from build123d import *

# Parameters (mm, degrees)
CROQUIS1_W              = 102
CROQUIS1_H              = 50
SALIENTE_EXTRUIR1_DEPTH = 40
CORTAR_EXTRUIR1_DEPTH   = 38
CROQUIS4_R              = 2
CORTAR_EXTRUIR2_DEPTH   = 18
CORTAR_EXTRUIR3_DEPTH   = 38
CROQUIS7_W              = 6
CROQUIS7_H              = 3
CORTAR_EXTRUIR5_DEPTH   = 10
SALIENTE_EXTRUIR2_DEPTH = 5
CROQUIS9_W              = 6
CROQUIS9_H              = 1
SALIENTE_EXTRUIR3_DEPTH = 3
REDONDEO2_R             = 2
REDONDEO4_R             = 2
CROQUIS16_W             = 36.5
CROQUIS16_H             = 26.972151698
CORTAR_EXTRUIR13_DEPTH  = 5.5
CROQUIS17_W             = 40
CROQUIS17_H             = 30
CROQUIS17_W_2           = 36.5
CROQUIS17_H_2           = 26.972151698
SALIENTE_EXTRUIR7_DEPTH = 13.5
CROQUIS18_W             = 1.5
CROQUIS18_H             = 36.5
SALIENTE_EXTRUIR8_DEPTH = 27.5
CROQUIS19_R             = 11
CORTAR_EXTRUIR14_DEPTH  = 27.5
REDONDEO5_R             = 2


with BuildPart() as part:
    # Croquis1 → Saliente-Extruir1 (new body)
    with BuildSketch(Plane.XY):
        Rectangle(CROQUIS1_W, CROQUIS1_H)
    extrude(amount=SALIENTE_EXTRUIR1_DEPTH)

    # Croquis3 → Cortar-Extruir1 (cut)
    with BuildSketch(Plane.XY.offset(40)):
        with BuildLine():
            Line((51, 25), (41, 25))
            Line((41, 25), (41, 18))
            ThreePointArc((41, 18), (41.878679656, 15.878679656), (44, 15))
            Line((44, 15), (51, 15))
            Line((51, 15), (51, 25))
        make_face()
        with BuildLine():
            Line((41, -18), (41, -25))
            Line((41, -25), (51, -25))
            Line((51, -25), (51, -15))
            Line((51, -15), (44, -15))
            ThreePointArc((44, -15), (41.878679656, -15.878679656), (41, -18))
        make_face()
        with BuildLine():
            Line((-44, -15), (-51, -15))
            Line((-51, -15), (-51, -25))
            Line((-51, -25), (-41, -25))
            Line((-41, -25), (-41, -18))
            ThreePointArc((-41, -18), (-41.878679656, -15.878679656), (-44, -15))
        make_face()
        with BuildLine():
            Line((-51, 25), (-51, 15))
            Line((-51, 15), (-44, 15))
            ThreePointArc((-44, 15), (-41.878679656, 15.878679656), (-41, 18))
            Line((-41, 18), (-41, 25))
            Line((-41, 25), (-51, 25))
        make_face()
    extrude(amount=-CORTAR_EXTRUIR1_DEPTH, mode=Mode.SUBTRACT)

    # Croquis4 → Cortar-Extruir2 (cut)
    with BuildSketch(Plane.XY.offset(2)):
        with BuildLine():
            Line((-51, -25), (-48, -25))
            ThreePointArc((-48, -25), (-50.121320344, -24.121320344), (-51, -22))
            Line((-51, -22), (-51, -25))
        make_face()
        with Locations((-46, -20)):
            Circle(CROQUIS4_R)
        with BuildLine():
            Line((-51, 25), (-51, 22))
            ThreePointArc((-51, 22), (-50.121320344, 24.121320344), (-48, 25))
            Line((-48, 25), (-51, 25))
        make_face()
        with Locations((-46, 20)):
            Circle(CROQUIS4_R)
        with Locations((46, 20)):
            Circle(CROQUIS4_R)
        with BuildLine():
            ThreePointArc((48, 25), (50.121320344, 24.121320344), (51, 22))
            Line((51, 22), (51, 25))
            Line((51, 25), (48, 25))
        make_face()
        with Locations((46, -20)):
            Circle(CROQUIS4_R)
        with BuildLine():
            ThreePointArc((51, -22), (50.121320344, -24.121320344), (48, -25))
            Line((48, -25), (51, -25))
            Line((51, -25), (51, -22))
        make_face()
    extrude(amount=-CORTAR_EXTRUIR2_DEPTH, mode=Mode.SUBTRACT)

    # Croquis5 → Cortar-Extruir3 (cut)
    with BuildSketch(Plane(origin=(0, 0, 0), x_dir=(-1, 0, 0), z_dir=(0, 0, -1))):
        with BuildLine():
            Line((0, 23.5), (-39.490487895, 23.5))
            Line((-39.490487895, 23.5), (-39.490487895, 15.5))
            ThreePointArc((-39.490487895, 15.5), (-40.076274332, 14.085786438), (-41.490487895, 13.5))
            Line((-41.490487895, 13.5), (-49.525351845, 13.5))
            Line((-49.525351845, 13.5), (-49.525351845, -13.472151698))
            Line((-49.525351845, -13.472151698), (-41.490487895, -13.472151698))
            ThreePointArc((-41.490487895, -13.472151698), (-40.076274332, -14.057938136), (-39.490487895, -15.472151698))
            Line((-39.490487895, -15.472151698), (-39.490487895, -23.5))
            Line((-39.490487895, -23.5), (39.5, -23.5))
            Line((39.5, -23.5), (39.5, -15.472151698))
            ThreePointArc((39.5, -15.472151698), (40.085786438, -14.057938136), (41.5, -13.472151698))
            Line((41.5, -13.472151698), (49.474648155, -13.472151698))
            Line((49.474648155, -13.472151698), (49.474648155, 13.5))
            Line((49.474648155, 13.5), (41.5, 13.5))
            ThreePointArc((41.5, 13.5), (40.085786438, 14.085786438), (39.5, 15.5))
            Line((39.5, 15.5), (39.5, 23.5))
            Line((39.5, 23.5), (0, 23.5))
        make_face()
    extrude(amount=-CORTAR_EXTRUIR3_DEPTH, mode=Mode.SUBTRACT)

    # Croquis7 → Cortar-Extruir5 (cut)
    with BuildSketch(Plane(origin=(0, 25, 0), x_dir=(1, 0, 0), z_dir=(0, 1, 0))):
        with Locations((0, -1.5)):
            Rectangle(CROQUIS7_W, CROQUIS7_H)
    extrude(amount=-CORTAR_EXTRUIR5_DEPTH, mode=Mode.SUBTRACT)

    # Croquis8 → Saliente-Extruir2 (add)
    with BuildSketch(Plane(origin=(0, 25, 0), x_dir=(1, 0, 0), z_dir=(0, 1, 0))):
        Polygon((3, 0), (4, 0), (4, -4), (-4, -4), (-4, 0), (-3, 0), (-3, -3), (3, -3), align=None)
    extrude(amount=SALIENTE_EXTRUIR2_DEPTH)

    # Croquis9 → Saliente-Extruir3 (add)
    with BuildSketch(Plane(origin=(0, 0, 3), x_dir=(-1, 0, 0), z_dir=(0, 0, -1))):
        with Locations((0, 29.5)):
            Rectangle(CROQUIS9_W, CROQUIS9_H)
    extrude(amount=SALIENTE_EXTRUIR3_DEPTH)

    # Redondeo2
    redondeo2_edges = [part.edges().sort_by_distance(p)[0] for p in [
        (0, 23.5, 3),
    ]]
    fillet(redondeo2_edges, radius=REDONDEO2_R)

    # Redondeo4
    redondeo4_edges = [part.edges().sort_by_distance(p)[0] for p in [
        (-4, 25, 2),
        (0, 25, 4),
        (4, 25, 2),
    ]]
    fillet(redondeo4_edges, radius=REDONDEO4_R)

    # Croquis16 → Cortar-Extruir13 (cut)
    with BuildSketch(Plane(origin=(-49.474648155, 0, 0), x_dir=(0, 0, -1), z_dir=(1, 0, 0))):
        with Locations((-19.75, 0.013924151)):
            Rectangle(CROQUIS16_W, CROQUIS16_H)
    extrude(amount=-CORTAR_EXTRUIR13_DEPTH, mode=Mode.SUBTRACT)

    # Croquis17 → Saliente-Extruir7 (add)
    with BuildSketch(Plane.ZY.offset(51)):
        with Locations((20, 0)):
            Rectangle(CROQUIS17_W, CROQUIS17_H)
        with Locations((19.75, 0.013924151)):
            Rectangle(CROQUIS17_W_2, CROQUIS17_H_2, mode=Mode.SUBTRACT)
    extrude(amount=SALIENTE_EXTRUIR7_DEPTH)

    # Croquis18 → Saliente-Extruir8 (add)
    with BuildSketch(Plane.XZ.offset(-13.5)):
        with Locations((-63.75, 19.75)):
            Rectangle(CROQUIS18_W, CROQUIS18_H)
    extrude(amount=SALIENTE_EXTRUIR8_DEPTH)

    # Croquis19 → Cortar-Extruir14 (cut)
    with BuildSketch(Plane.ZY.offset(64.5)):
        with Locations((20, 0)):
            Circle(CROQUIS19_R)
    extrude(amount=-CORTAR_EXTRUIR14_DEPTH, mode=Mode.SUBTRACT)

    # Redondeo5
    redondeo5_edges = [part.edges().sort_by_distance(p)[0] for p in [
        (51, 0, 40),
        (0, 25, 40),
        (0, -25, 40),
        (-41.878679656, 15.878679656, 40),
        (-41, 21.5, 40),
        (-64.5, 0, 40),
        (-54.25, 15, 40),
        (-41.878679656, -15.878679656, 40),
        (-41, -21.5, 40),
        (-54.25, -15, 40),
        (41.878679656, -15.878679656, 40),
        (47.5, -15, 40),
        (41, -21.5, 40),
        (41.878679656, 15.878679656, 40),
        (47.5, 15, 40),
        (41, 21.5, 40),
    ]]
    fillet(redondeo5_edges, radius=REDONDEO5_R)


solid = part.part
Check sheet for the modelled part. Datum: model origin and axes. Units: mm. A direction names the side the tool comes from. Round coordinates to 2 decimals unless told otherwise and drop trailing zeros. Order: outer loops, then holes, each group sorted by start corner. A loop starts at its lowest first (then second) coordinate and runs counter-clockwise, first axis right, second up. Notation, with made-up numbers: M 9.5,45.25 L 32.5,45.25 A32 cw 32.5,74.25 Z; hole C -24,13 d8. An arc over 180 degrees is marked long. One line per item, written item: value. Start each with the question number.
1. Section check C-C on y = 20. Enter the section's corners in (x, z).
2. Section check D-D on x = 35. Enter the section's corners in (y, z).
3. Release check for a two-part mould opening along Z. For faces 6 (the flat face through (-43.8, 20.1, 2)), 7 (the flat face through (51, 0, 19)), 8 (the flat face through (-52, -13.472, 19)) record: released by +Z, released by -Z, zero draft, split by the parting line, or undercut.
4. Section check B-B on y = 0. Enter the section's corners in (x, z).
5. Access from +Z, -Z, +X, -X, +Y, -Y to the whole of each face (thin tool, end or side, straight path). Record for faces 1 (the flat face through (-63, -12, 19)), 2 (the flat face through (0, 27, 3)), 3 (the flat face through (48.2, -19.9, 2)), 4 (the cylindrical face through (-41.9, 15.86, 20.25)), 5 (the cylindrical face through (41.86, 15.9, 20.25)).
6. Gauge pin test, flat ends, axial feed: P1, Ø0.9, axis at x = 2, y = 28.5, coming from the +Z side; P2, Ø4, axis at y = 18.5, z = 14.5, coming from the +X side; P3, Ø5.5, axis at y = -22.5, z = 22, coming from the -X side. Record the tip position at first contact, or that the pin passes through.
7. Section check A-A on x = -46. Enter the section's corners in (y, z), and give its area (3 significant figures).
8. Scan lines: line 1 along Y through (x, z) = (-46, 1); line 2 along Y through (x, z) = (-8.5, 7); line 3 along Y through (x, z) = (-58, 6). Record each from-to range of solid material in increasing order.
Results found:
1. outline: M -51,0 L -48,0 L -48,2 L -51,2 Z; M -44,0 L -39.5,0 L -39.5,38 L 39.49,38 L 39.49,0 L 44,0 L 44,2 L 41,2 L 41,38 A2 ccw 39,40 L -39,40 A2 ccw -41,38 L -41,2 L -44,2 Z; M 48,0 L 51,0 L 51,2 L 48,2 Z
2. outline: M -25,0 L -23.5,0 L -23.5,38 L 23.5,38 L 23.5,0 L 25,0 L 25,38 A2 ccw 23,40 L -23,40 A2 ccw -25,38 Z
3. face 6: released by +Z
3. face 7: zero draft
3. face 8: undercut
4. outline: M -64.5,0 L -49.47,0 L -49.47,1.5 L -63,1.5 L -63,9 L -64.5,9 Z; M -64.5,31 L -63,31 L -63,38 L 49.53,38 L 49.53,0 L 51,0 L 51,38 A2 ccw 49,40 L -62.5,40 A2 ccw -64.5,38 Z
5. face 1: none
5. face 2: -Z
5. face 3: +Z, +X, -Y
5. face 4: +Z, -X, +Y
5. face 5: +Z, +X, +Y
6. P1: z = 4
6. P2: x = 41.4
6. P3: x = -41
7. outline: M -25,0 L -22,0 L -22,2 L -25,2 Z; M -18,0 L -13.47,0 L -13.47,38 L 13.5,38 L 13.5,0 L 18,0 L 18,2 L 15,2 L 15,38 A2 ccw 13,40 L -13,40 A2 ccw -15,38 L -15,2 L -18,2 Z; M 22,0 L 25,0 L 25,2 L 22,2 Z
7. area: 197 mm^2
8. line 1: -25 to -22, -18 to -13.47, 13.5 to 18, 22 to 25
8. line 2: -25 to -23.5, 23.5 to 25
8. line 3: -15 to -13.47, 13.5 to 15
